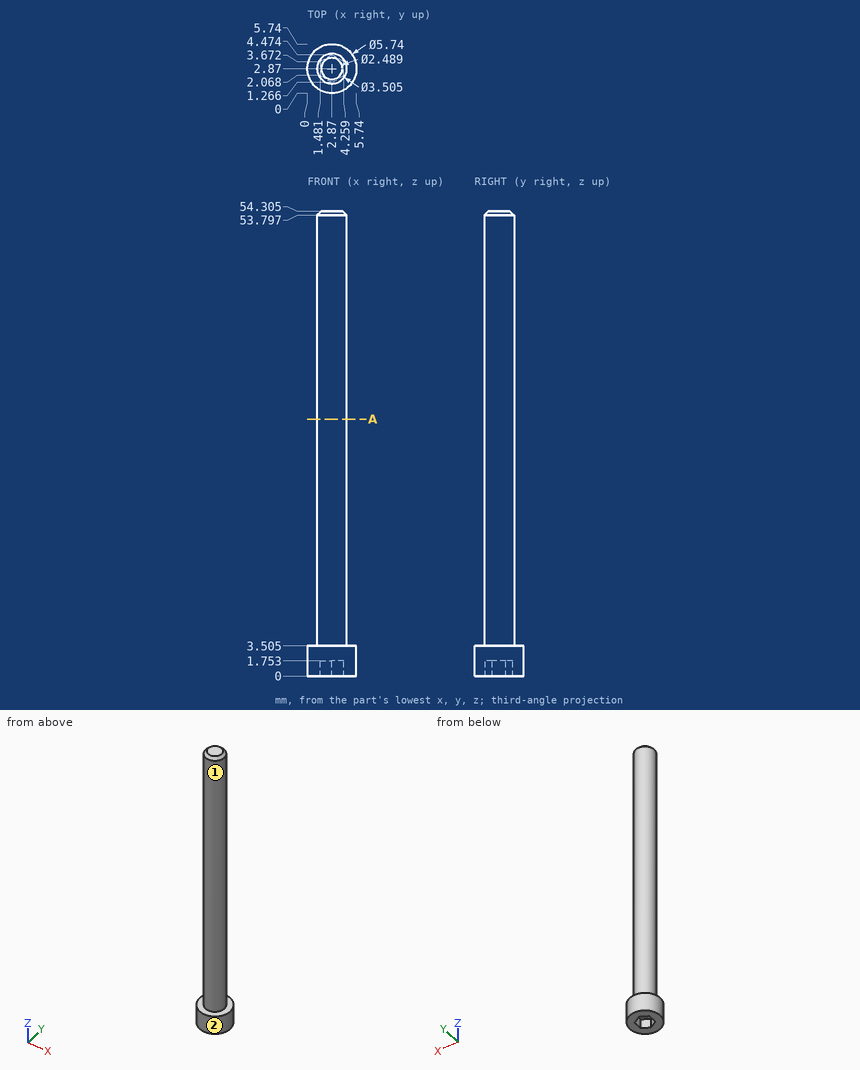
Here's the drawing with two shaded views (mm, measured from the low corner). I have some questions. A direction names the side the tool comes from. Coordinates: 2 decimals unless noted, no trailing zeros. Loops run counter-clockwise (first coordinate to the right, second up) from the corner with the lowest first, then second, coordinate; pieces in that order, holes last. Notation, with made-up numbers: (19, 68) -> (27, 68) arc R9 cw to (27, 73) -> close; hole circle Ø1 at (18.25, 7.25). An arc over 180 degrees is marked (long way). Answer in a Markdown table with one row per item.
(1) Will these pins go through, and if not, where does the flat tip stop? pin 1 Ø0.8 at (y, z) = (3, 0.5) entering from +X; pin 2 Ø1 at (x, z) = (4, 43) entering from -Y (1 decimal); pin 3 Ø1.4 at (x, y) = (3.5, 2.5) entering from -Z; pin 4 Ø1 at (y, z) = (3, 45.5) entering from +X.
Results found:
| item | result |
|---|---|
| pin 1 | stops at x = 5.74 |
| pin 2 | stops at y = 1.2 |
| pin 3 | stops at z = 1.75 |
| pin 4 | stops at x = 4.62 |
(2) For the marked faces 1 and 2, which set-ups out of +Z, -Z, +X, -X, +Y, -Y let a thin tool reach every point of the face, with its end or its side?
Results found:
| item | result |
|---|---|
| face 1 | +Z |
| face 2 | +Z, -Z |
(3) If I drill on probe 1 along Y at (x, z) = (3.05, 32.5); probe 2 along Z at (x, y) = (1.8, 1.25) (1 decimal); probe 3 along Z at (x, y) = (2.55, 3.45) (1 decimal), over which ranges is the centre line in solid material (lowest first)?
Results found:
| item | result |
|---|---|
| probe 1 | y = 1.13 to 4.61 |
| probe 2 | z = 0 to 3.5 |
| probe 3 | z = 1.8 to 54.3 |
(4) Imagine slicing it at A-A (z = 30). List the corners of the cut face in (x, y) for me (1 decimal).
Results found:
| item | result |
|---|---|
| outline | circle Ø3.5 at (2.9, 2.9) |
